Read the model definition and answer for the solid it produces. Units are mm, in the model's axes. A direction names the side the tool comes from. Coordinates: 2 decimals unless noted, no trailing zeros. Write each loop counter-clockwise with the first axis right and the second up, starting at its lowest first coordinate (ties: lowest second). Pieces come first, ordered by that corner, then holes. Notation, with made-up numbers: (52.25, 54.25) -> (102.25, 54.25) arc R26 cw to (102.25, 82.25) -> close; hole circle Ø7 at (67, 79.5). An arc over 180 degrees is marked (long way). Write item = value, one per line. Start each with the question number.
1) Section A-A (x = -31) is taken. Determine the outline of the cut face in (y, z).
2) A tool of negligible diameter and unlimited length cuts with its end or side. For faces 5 (the face through (-47.019, -49, -21)), 6 (the face through (-34.319, -49, -21)), 7 (the face through (-58.27, -12.88, -38.86)), from which of +Z, -Z, +X, -X, +Y, -Y can it reach the whole face along a straight path? Write none if from no direction.
3) Section C-C (x = -42) is taken. Determine the outline of the cut face in (y, z).
4) Find the intervals of material crossed by line 1 along Y through (x, z) = (-2.5, -24); line 2 along Z through (x, y) = (-41, -50); line 3 along X through (y, z) = (-14, -20.5), in increasing order. Write a range as from..to.
5) For a pull along Z with two mould halves and no side action, classify faces 1 (the face through (-41, -50, -27.687)), 2 (the face through (-41, -50, -14.987)), 3 (the face through (-29.28, -12.52, 31.95)), 4 (the face through (-35.044, -75.436, -21.248)) as released by +Z, released by -Z, zero draft, split by the parting line, or undercut.
6) Section B-B (z = -10.5) is taken. Determine the outline of the cut face in (x, y), plus the area to 3 significant figures.
7) Flat-ended cylindrical pins translate along their axes: pin 1 Ø4 at (x, y) = (-40, -39.5) entering from +Z; pin 2 Ø14.5 at (x, z) = (16.48, -14.99) entering from -Y; pin 3 Ø4 at (x, y) = (-37.5, -46.5) entering from -Z. Find the tip coordinate at first contact, or state that the pin passes through.
8) Section D-D (y = -42.5) is taken. Determine the outline of the cut face in (x, z).
from build123d import *

# Parameters (mm, degrees)
F0_W      = 101.6
F0_H      = 101.6
F1_DEPTH  = 25.4
F2_R      = 5.08
F3_R      = 5.08
F4_R      = 5.08
F5_R      = 5.08
F8_D      = 12.7
F10_W     = 12.7
F10_H     = 12.7
F11_DEPTH = 50.8
F12_R     = 2.54
F13_R     = 2.54


with BuildPart() as f1:
    # F0 (on Front) → F1 (new body)
    with BuildSketch(Plane.XZ):
        with Locations((-8.919485, 10.413215)):
            Rectangle(F0_W, F0_H)
    extrude(amount=F1_DEPTH)

    # F2
    f2_edges = [f1.edges().sort_by_distance(p)[0] for p in [
        (-59.719485, -12.7, 61.213215),
    ]]
    fillet(f2_edges, radius=F2_R)

    # F3
    f3_edges = [f1.edges().sort_by_distance(p)[0] for p in [
        (-59.719485, -12.7, -40.386785),
    ]]
    fillet(f3_edges, radius=F3_R)

    # F4
    f4_edges = [f1.edges().sort_by_distance(p)[0] for p in [
        (41.880515, -12.7, -40.386785),
    ]]
    fillet(f4_edges, radius=F4_R)

    # F5
    f5_edges = [f1.edges().sort_by_distance(p)[0] for p in [
        (41.880515, -12.7, 61.213215),
    ]]
    fillet(f5_edges, radius=F5_R)

    # F8 (through all)
    with Locations(Plane.XZ.offset(25.4)):
        with Locations((-34.319485, 35.813215), (16.480515, -14.986785)):
            Hole(F8_D / 2)

    # F10 (on face) → F11 (join)
    with BuildSketch(Plane.XZ.offset(25.4)):
        with Locations((-40.669485, -21.336785)):
            Rectangle(F10_W, F10_H)
    extrude(amount=F11_DEPTH)

    # F12
    f12_edges = [f1.edges().sort_by_distance(p)[0] for p in [
        (-34.319485, -76.2, -21.336785),
    ]]
    fillet(f12_edges, radius=F12_R)

    # F13
    f13_edges = [f1.edges().sort_by_distance(p)[0] for p in [
        (-47.019485, -76.2, -21.336785),
    ]]
    fillet(f13_edges, radius=F13_R)


solid = f1.part
Answer key:
q1.outline = (-25.4, -40.39) -> (0, -40.39) -> (0, 30.4) -> (-25.4, 30.4) -> close; (-25.4, 41.23) -> (0, 41.23) -> (0, 61.21) -> (-25.4, 61.21) -> close
q2.face_5 = +Z, -Z, -X, -Y
q2.face_6 = +Z, -Z, +X, -Y
q2.face_7 = -Z, -X, +Y, -Y
q3.outline = (-76.2, -27.69) -> (-25.4, -27.69) -> (-25.4, -40.39) -> (0, -40.39) -> (0, 61.21) -> (-25.4, 61.21) -> (-25.4, -14.99) -> (-76.2, -14.99) -> close
q4.line_1 = -25.4..0
q4.line_2 = -27.69..-14.99
q4.line_3 = -59.72..13.33, 19.63..41.88
q5.face_1 = released by -Z
q5.face_2 = released by +Z
q5.face_3 = undercut
q5.face_4 = zero draft
q6.outline = (-59.72, -25.4) -> (11.99, -25.4) -> (11.99, 0) -> (-59.72, 0) -> close; (20.97, -25.4) -> (41.88, -25.4) -> (41.88, 0) -> (20.97, 0) -> close
q6.area = 2,350 mm^2
q7.pin_1 = -14.99
q7.pin_2 = -25.4
q7.pin_3 = -27.69
q8.outline = (-47.02, -27.69) -> (-34.32, -27.69) -> (-34.32, -14.99) -> (-47.02, -14.99) -> close
